from build123d import *

# Parameters (mm, degrees)
SALIENTE_EXTRUIR1_DEPTH      = 27.5
SALIENTE_EXTRUIR1_DEPTH_BACK = 27.5
CROQUIS2_R                   = 4
CORTAR_EXTRUIR1_DEPTH        = 30
CROQUIS3_R                   = 2.5
CORTAR_EXTRUIR2_DEPTH        = 22
CORTAR_EXTRUIR3_START        = -22
CROQUIS4_R                   = 2.5
CORTAR_EXTRUIR3_DEPTH        = 22
CROQUIS5_R                   = 11
CORTAR_EXTRUIR4_DEPTH        = 2
CROQUIS6_R                   = 5.75
CORTAR_EXTRUIR5_DEPTH        = 20
CORTAR_EXTRUIR6_START        = -20
CROQUIS7_R                   = 5.75
CORTAR_EXTRUIR6_DEPTH        = 20
CROQUIS8_R                   = 3
CORTAR_EXTRUIR7_DEPTH        = 30


with BuildPart() as part:
    # Croquis1 → Saliente-Extruir1 (new, two sides: drawn at the far end of the back side and taken through both)
    with BuildSketch(Plane.XY.offset(-SALIENTE_EXTRUIR1_DEPTH_BACK)):
        Polygon((37.5, 0), (-37.5, 0), (-37.5, -35), (-27.5, -35), (-27.5, -112), (27.5, -112), (27.5, -35), (37.5, -35), align=None)
    extrude(amount=SALIENTE_EXTRUIR1_DEPTH + SALIENTE_EXTRUIR1_DEPTH_BACK)

    # Croquis2 → Cortar-Extruir1 (cut)
    with BuildSketch(Plane(origin=(0, 0, 0), x_dir=(1, 0, 0), z_dir=(0, 1, 0))):
        with Locations(Location((-30, 0, 0), (0, 0, 180))):
            Circle(CROQUIS2_R)
        with Locations(Location((0, 20, 0), (0, 0, 180))):
            Circle(CROQUIS2_R)
        with Locations(Location((30, 0, 0), (0, 0, 180))):
            Circle(CROQUIS2_R)
        with Locations(Location((0, -20, 0), (0, 0, 180))):
            Circle(CROQUIS2_R)
    extrude(amount=-CORTAR_EXTRUIR1_DEPTH, mode=Mode.SUBTRACT)

    # Croquis3 → Cortar-Extruir2 (cut)
    with BuildSketch(Plane(origin=(27.5, 0, 0), x_dir=(0, 0, -1), z_dir=(1, 0, 0))):
        with Locations(Location((-21.5, -94, 0), (0, 0, 90))):
            Circle(CROQUIS3_R)
        with Locations(Location((-21.5, -72, 0), (0, 0, 90))):
            Circle(CROQUIS3_R)
        with Locations(Location((21.5, -72, 0), (0, 0, 90))):
            Circle(CROQUIS3_R)
        with Locations(Location((21.5, -94, 0), (0, 0, 90))):
            Circle(CROQUIS3_R)
    extrude(amount=-CORTAR_EXTRUIR2_DEPTH, mode=Mode.SUBTRACT)

    # Croquis4 → Cortar-Extruir3 (cut)
    with BuildSketch(Plane.ZY.offset(27.5).offset(CORTAR_EXTRUIR3_START)):
        with Locations(Location((-21.5, -94, 0), (0, 0, 90))):
            Circle(CROQUIS4_R)
        with Locations(Location((-21.5, -72, 0), (0, 0, 90))):
            Circle(CROQUIS4_R)
        with Locations(Location((21.5, -72, 0), (0, 0, 90))):
            Circle(CROQUIS4_R)
        with Locations(Location((21.5, -94, 0), (0, 0, 90))):
            Circle(CROQUIS4_R)
    extrude(amount=CORTAR_EXTRUIR3_DEPTH, mode=Mode.SUBTRACT)

    # Croquis5 → Cortar-Extruir4 (cut)
    with BuildSketch(Plane.XZ.offset(112)):
        with Locations(Location((0, 0, 0), (0, 0, 270))):
            Circle(CROQUIS5_R)
    extrude(amount=-CORTAR_EXTRUIR4_DEPTH, mode=Mode.SUBTRACT)

    # Croquis6 → Cortar-Extruir5 (cut)
    with BuildSketch(Plane(origin=(37.5, 0, 0), x_dir=(0, 0, -1), z_dir=(1, 0, 0))):
        with Locations((13, -20)):
            Circle(CROQUIS6_R)
    extrude(amount=-CORTAR_EXTRUIR5_DEPTH, mode=Mode.SUBTRACT)

    # Croquis7 → Cortar-Extruir6 (cut)
    with BuildSketch(Plane.ZY.offset(37.5).offset(CORTAR_EXTRUIR6_START)):
        with Locations(Location((-13, -20, 0), (0, 0, 180))):
            Circle(CROQUIS7_R)
    extrude(amount=CORTAR_EXTRUIR6_DEPTH, mode=Mode.SUBTRACT)

    # Croquis8 → Cortar-Extruir7 (cut)
    with BuildSketch(Plane.XZ.offset(110)):
        with Locations(Location((0, 0, 0), (0, 0, 270))):
            Circle(CROQUIS8_R)
    extrude(amount=-CORTAR_EXTRUIR7_DEPTH, mode=Mode.SUBTRACT)


solid = part.part
Here's how the part is built. I have some questions about the finished solid (model axes, mm). A direction names the side the tool comes from. Coordinates: 2 decimals unless noted, no trailing zeros. Write each loop counter-clockwise with the first axis right and the second up, starting at its lowest first coordinate (ties: lowest second). Pieces come first, ordered by that corner, then holes.
1) Thinking about a two-plate mould opening in Y: for faces 6 (the face through (-16.3, -96.5, 21.4)), 7 (the face through (-26.8, -14.8, -2.4)), 8 (the face through (-16, -96, -23)), 9 (the face through (0, -30, -20)), which applies, +Y half, -Y half, draft (parallel to the pull), parting line (faces both ways), or undercut?
Filled in:
face 6: undercut
face 7: draft
face 8: undercut
face 9: +Y half
2) If we section it at A-A (y = -94): List the corners of the cut face in (x, z) for me, plus the area to 3 significant figures.
Filled in:
outline: (-27.5, -27.5) - (27.5, -27.5) - (27.5, -24) - (5.5, -24) - (5.5, -19) - (27.5, -19) - (27.5, 19) - (5.5, 19) - (5.5, 24) - (27.5, 24) - (27.5, 27.5) - (-27.5, 27.5) - (-27.5, 24) - (-5.5, 24) - (-5.5, 19) - (-27.5, 19) - (-27.5, -19) - (-5.5, -19) - (-5.5, -24) - (-27.5, -24) - close; hole circle Ø6 at (0, 0)
area: 2,560 mm2
3) If I drill on line 1 (Y direction, x = 28, z = -13); line 2 (Y direction, x = -19, z = -22); line 3 (X direction, y = -94, z = 0), over which ranges is the centre line in solid material (lowest first)?
Filled in:
line 1: y = -35 to -25.75, -14.25 to 0
line 2: y = -112 to -96.45, -91.55 to -74.45, -69.55 to 0
line 3: x = -27.5 to -3, 3 to 27.5
4) Which directions (+Z, -Z, +X, -X, +Y, -Y) give clear straight access to the entire face, cutting with the end or side of a thin tool? Please do faces 1 (the face through (30, -30, 0)), 2 (the face through (-33, -35, 0)), 3 (the face through (5.5, -94, 22)), 4 (the face through (27.5, -74, 0)), 5 (the face through (-27.36, -14.899, -15.653)).
Filled in:
face 1: +Y
face 2: +Z, -Z, -X, -Y
face 3: +X
face 4: +Z, -Z, +X, -Y
face 5: -X
5) If we section it at C-C (y = -72): List the corners of the cut face in (x, z) for me, plus the area to 4 significant figures.
Filled in:
outline: (-27.5, -27.5) - (27.5, -27.5) - (27.5, -24) - (5.5, -24) - (5.5, -19) - (27.5, -19) - (27.5, 19) - (5.5, 19) - (5.5, 24) - (27.5, 24) - (27.5, 27.5) - (-27.5, 27.5) - (-27.5, 24) - (-5.5, 24) - (-5.5, 19) - (-27.5, 19) - (-27.5, -19) - (-5.5, -19) - (-5.5, -24) - (-27.5, -24) - close
area: 2,585 mm2
6) If we section it at D-D (x = -19): List the corners of the cut face in (y, z) for me.
Filled in:
outline: (-112, -27.5) - (0, -27.5) - (0, 27.5) - (-112, 27.5) - close; hole circle Ø5 at (-94, -21.5); hole circle Ø5 at (-94, 21.5); hole circle Ø5 at (-72, -21.5); hole circle Ø5 at (-72, 21.5); hole circle Ø11.5 at (-20, -13)
7) If we section it at B-B (x = -30): List the corners of the cut face in (y, z) for me.
Filled in:
outline: (-35, -27.5) - (0, -27.5) - (0, -4) - (-30, -4) - (-30, 4) - (0, 4) - (0, 27.5) - (-35, 27.5) - close; hole circle Ø11.5 at (-20, -13)
8) I'm going to push flat-ended pins straight in: pin 1 (1.5 mm diameter, centred on y = -71.5, z = 22, fed in from -X); pin 2 (3.5 mm diameter, centred on x = 0, z = 0, fed in from +Y); pin 3 (1 mm diameter, centred on y = -80.5, z = 2.5, fed in from -X); pin 4 (4.5 mm diameter, centred on y = -72, z = 21.5, fed in from +X). Where does each tip first touch, or does it pass through?
Filled in:
pin 1: stops at x = -5.5
pin 2: stops at y = 0
pin 3: stops at x = -27.5
pin 4: stops at x = 5.5
